Study the drawing (mm; zero at the part's minimum x, y, z) and answer. Round coordinates to 2 decimals unless told otherwise and drop trailing zeros. Order: outer loops, then holes, each group sorted by start corner. A loop starts at its lowest first (then second) coordinate and runs counter-clockwise, first axis right, second up. Notation, with made-up numbers: M -13.5,47.25 L 45.5,47.25 A20 cw 45.5,71.25 Z; hole C -16.75,0 d3. An arc over 180 degrees is marked long. Put each result on its own line as item: value. Start each with the question number.
1. This flat-tipped pin is pushed along its axis until it touches: pin 1 Ø2 at (x, z) = (13, 12.5) entering from -Y. Where does it stop, or does it pass through?
2. Consider line 1 (X direction, y = 0.65, z = 17.5); line 2 (Z direction, x = 46, y = 1.15) (1 decimal); line 3 (X direction, y = 0.8, z = 29) (1 decimal). Determine where each line is inside the solid, lowest interval first.
3. The part is cut by section A-A (y = 1.15). Count the separate pieces of the cut face and the enclosed holes in it, then the cut area to 3 significant figures.
4. The part is cut by section B-B (z = 34.5). Give the vertices of the cut face in (x, y).
5. The part is cut by section C-C (z = 20.5). Give the vertices of the cut face in (x, y) (1 decimal).
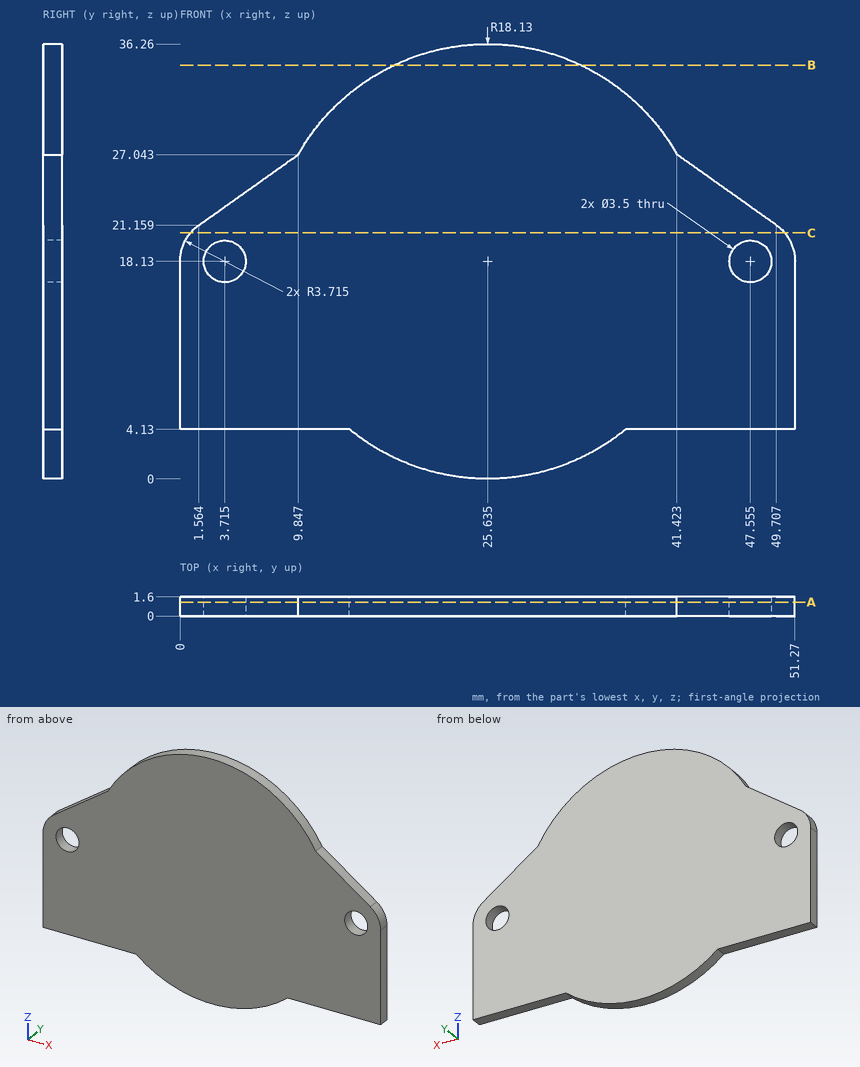
Resolved:
1. pin 1: y = 0
2. line 1: 0 to 2.08, 5.35 to 45.92, 49.19 to 51.27
2. line 2: 4.1 to 17.3, 18.9 to 23.8
2. line 3: 11.1 to 40.1
3. separate pieces: 1
3. enclosed holes: 2
3. area: 1,360 mm2
4. outline: M 17.84,0 L 33.43,0 L 33.43,1.6 L 17.84,1.6 Z
5. outline: M 0.9,0 L 50.4,0 L 50.4,1.6 L 0.9,1.6 Z
